For this review, take the finished solid that the model builds, in its own axes (mm). Face numbers are marked on the shaded views. A direction names the side the tool comes from. Coordinates: 2 decimals unless noted, no trailing zeros. Loops run counter-clockwise (first coordinate to the right, second up) from the corner with the lowest first, then second, coordinate; pieces in that order, holes last.
1. Mouldability with a two-part tool opening along X and no side actions: class the marked faces 4, 5, 6 and 7 as pulls with the +X half, pulls with the -X half, needs draft (parallel to the pull), parting line crosses it, or undercut.
2. Take a section at B-B, the plane z = -15.25. State the section outline as (x, y) points, then the cut area to 3 significant figures.
3. To check wall thickness, follow probe 1 along X at (y, z) = (0, -12); probe 2 along Z at (x, y) = (10.5, 2.25). State the ranges of each line that lie inside material, in increasing order.
4. Take a section at C-C, the plane y = -2.5. Count the separate pieces of the cut face and the enclosed holes in it, then the cut area to 3 significant figures.
5. Take a section at D-D, the plane z = -6. State the section outline as (x, y) points.
6. Take a section at A-A, the plane x = 0. State the section outline as (y, z) points.
7. Clearance check with flat-ended pins moving along their axes: P1, Ø3, axis at y = 6.5, z = -10, coming from the +X side; P2, Ø0.8, axis at x = 7, z = -9, coming from the +Y side; P3, Ø8, axis at x = 0, y = 0, coming from the +Z side. State where each tip first meets the part, or that it passes through.
8. Machinability: for the marked faces 1, 2 and 3, which of the approach directions +Z, -Z, +X, -X, +Y, -Y give a long, thin tool a straight path to every point of the face, cutting with its end or side? Answer none if there is none.
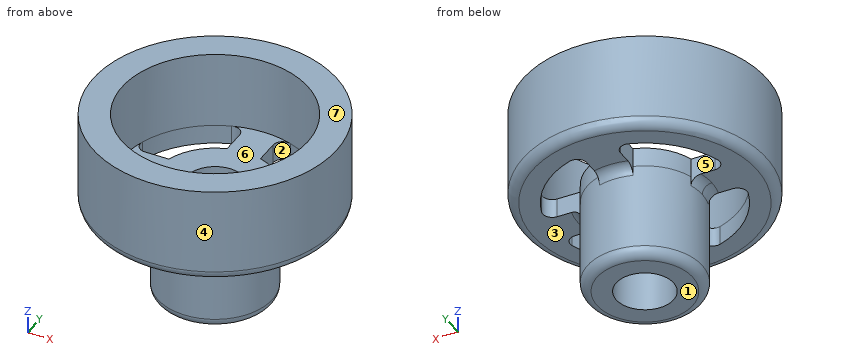
```python
from build123d import *
from build123d.topology import SkipClean

# Parameters (mm, degrees)
ESBO_O1_R                = 12.7
ESBO_O1_R_2              = 9.7
ESBO_O1_R_3              = 3
RESSALTO_EXTRUS_O1_DEPTH = 10
ESBO_O1_3_R              = 9.7
ESBO_O1_3_R_2            = 3
CORTE_EXTRUS_O1_DEPTH    = 8
CORTE_EXTRUS_O3_START    = -2
CORTE_EXTRUS_O3_DEPTH    = 2
FILETE1_R                = 1
ESBO_O2_5_R              = 6
ESBO_O2_5_R_2            = 3
RESSALTO_EXTRUS_O2_DEPTH = 10
FILETE2_R                = 1
FILETE3_R                = 1
FILETE4_R                = 1


with BuildPart() as part:
    # Esboço1 → Ressalto-extrusão1 (new body)
    # profile 1 of 2: a face of its own
    with BuildSketch(Plane.XY):
        Circle(ESBO_O1_R)
        Circle(ESBO_O1_R_2, mode=Mode.SUBTRACT)
    # profile 2 of 2: a face of its own
    with BuildSketch(Plane.XY):
        Circle(ESBO_O1_R_2)
        Circle(ESBO_O1_R_3, mode=Mode.SUBTRACT)
    extrude(amount=-RESSALTO_EXTRUS_O1_DEPTH)

    # Esboço1<3> → Corte-extrusão1 (cut)
    with BuildSketch(Plane.XY):
        Circle(ESBO_O1_3_R)
        Circle(ESBO_O1_3_R_2, mode=Mode.SUBTRACT)
    extrude(amount=-CORTE_EXTRUS_O1_DEPTH, mode=Mode.SUBTRACT)

    # Esboço2 → Corte-extrusão3 (cut)
    with SkipClean():  # the faces are left unmerged after this step: merging them gives an invalid solid
        with BuildSketch(Plane(origin=(0, 0, -10), x_dir=(-1, 0, 0), z_dir=(0, 0, -1)).offset(CORTE_EXTRUS_O3_START)):
            with BuildLine():
                Line((-1.75, -9.540833), (-1.75, -5.73912))
                ThreePointArc((-1.75, -5.73912), (-4.242641, -4.242641), (-5.73912, -1.75))
                Line((-5.73912, -1.75), (-9.540833, -1.75))
                ThreePointArc((-9.540833, -1.75), (-6.858936, -6.858936), (-1.75, -9.540833))
            make_face()
            with BuildLine():
                Line((-9.540833, 1.75), (-5.73912, 1.75))
                ThreePointArc((-5.73912, 1.75), (-4.242641, 4.242641), (-1.75, 5.73912))
                Line((-1.75, 5.73912), (-1.75, 9.540833))
                ThreePointArc((-1.75, 9.540833), (-6.858936, 6.858936), (-9.540833, 1.75))
            make_face()
            with BuildLine():
                Line((5.73912, 1.75), (9.540833, 1.75))
                ThreePointArc((9.540833, 1.75), (6.858936, 6.858936), (1.75, 9.540833))
                Line((1.75, 9.540833), (1.75, 5.73912))
                ThreePointArc((1.75, 5.73912), (4.242641, 4.242641), (5.73912, 1.75))
            make_face()
            with BuildLine():
                ThreePointArc((1.75, -9.540833), (6.858936, -6.858936), (9.540833, -1.75))
                Line((9.540833, -1.75), (5.73912, -1.75))
                ThreePointArc((5.73912, -1.75), (4.242641, -4.242641), (1.75, -5.73912))
                Line((1.75, -5.73912), (1.75, -9.540833))
            make_face()
        extrude(amount=CORTE_EXTRUS_O3_DEPTH, mode=Mode.SUBTRACT)

    # Filete1
    filete1_edges = [part.edges().sort_by_distance(p)[0] for p in [
        (-9.540833, -1.75, -9),
        (-1.75, -9.540833, -9),
        (-1.75, 9.540833, -9),
        (-9.540833, 1.75, -9),
        (9.540833, 1.75, -9),
        (1.75, 9.540833, -9),
        (1.75, -9.540833, -9),
        (9.540833, -1.75, -9),
    ]]
    fillet(filete1_edges, radius=FILETE1_R)

    # Esboço2<5> → Ressalto-extrusão2 (add)
    with SkipClean():  # the faces are left unmerged after this step: merging them gives an invalid solid
        with BuildSketch(Plane(origin=(0, 0, -10), x_dir=(-1, 0, 0), z_dir=(0, 0, -1))):
            Circle(ESBO_O2_5_R)
            with Locations(Location((0, 0, 0), (0, 0, 180))):
                Circle(ESBO_O2_5_R_2, mode=Mode.SUBTRACT)
        extrude(amount=RESSALTO_EXTRUS_O2_DEPTH)

    # Filete2
    # the kernel refuses this fillet: 1 mm, written as the material it adds along each edge
    with BuildSketch(Plane(origin=(0, 0, -10), x_dir=(-1, 0, 0), z_dir=(0, -1, 0))) as filete2_piece_1_section:
        with BuildLine():
            CenterArc((6 + FILETE2_R, FILETE2_R), FILETE2_R, 180, 90)
            Line((6, FILETE2_R), (6, 0))
            Line((6, 0), (6 + FILETE2_R, 0))
        make_face()
    filete2_piece_1 = revolve(axis=Axis((0, 0, -10), (0, 0, -1)), revolution_arc=40.831345, mode=Mode.PRIVATE)
    filete2_piece_1 = split(filete2_piece_1, bisect_by=Plane(origin=(-6.142197, 1.75, -10.226515), z_dir=(0, -1, 0)), keep=Keep.TOP, mode=Mode.PRIVATE)
    add(filete2_piece_1)
    with BuildSketch(Plane(origin=(0, 0, -10), x_dir=(0.6538481250913037, -0.7566258185619804, 0), z_dir=(0.7566258185619804, 0.6538481250913037, 0))) as filete2_piece_2_section:
        with BuildLine():
            CenterArc((6 + FILETE2_R, FILETE2_R), FILETE2_R, 180, 90)
            Line((6, FILETE2_R), (6, 0))
            Line((6, 0), (6 + FILETE2_R, 0))
        make_face()
    filete2_piece_2 = revolve(axis=Axis((0, 0, -10), (0, 0, -1)), revolution_arc=81.664733, mode=Mode.PRIVATE)
    filete2_piece_2 = split(filete2_piece_2, bisect_by=Plane(origin=(-1.75, -6.142197, -10.226515), z_dir=(1, 0, 0)), keep=Keep.TOP, mode=Mode.PRIVATE)
    filete2_piece_2 = split(filete2_piece_2, bisect_by=Plane(origin=(1.75, -6.142197, -10.226515), z_dir=(-1, 0, 0)), keep=Keep.TOP, mode=Mode.PRIVATE)
    add(filete2_piece_2)
    with BuildSketch(Plane(origin=(0, 0, -10), x_dir=(0.7566258185619548, 0.6538481250913332, 0), z_dir=(-0.6538481250913332, 0.7566258185619548, 0))) as filete2_piece_3_section:
        with BuildLine():
            CenterArc((6 + FILETE2_R, FILETE2_R), FILETE2_R, 180, 90)
            Line((6, FILETE2_R), (6, 0))
            Line((6, 0), (6 + FILETE2_R, 0))
        make_face()
    filete2_piece_3 = revolve(axis=Axis((0, 0, -10), (0, 0, -1)), revolution_arc=81.664733, mode=Mode.PRIVATE)
    filete2_piece_3 = split(filete2_piece_3, bisect_by=Plane(origin=(6.142197, -1.75, -10.226515), z_dir=(0, 1, 0)), keep=Keep.TOP, mode=Mode.PRIVATE)
    filete2_piece_3 = split(filete2_piece_3, bisect_by=Plane(origin=(6.142197, 1.75, -10.226515), z_dir=(0, -1, 0)), keep=Keep.TOP, mode=Mode.PRIVATE)
    add(filete2_piece_3)
    with BuildSketch(Plane(origin=(0, 0, -10), x_dir=(-0.6538481250913029, 0.7566258185619811, 0), z_dir=(-0.7566258185619811, -0.6538481250913029, 0))) as filete2_piece_4_section:
        with BuildLine():
            CenterArc((6 + FILETE2_R, FILETE2_R), FILETE2_R, 180, 90)
            Line((6, FILETE2_R), (6, 0))
            Line((6, 0), (6 + FILETE2_R, 0))
        make_face()
    filete2_piece_4 = revolve(axis=Axis((0, 0, -10), (0, 0, -1)), revolution_arc=81.664733, mode=Mode.PRIVATE)
    filete2_piece_4 = split(filete2_piece_4, bisect_by=Plane(origin=(1.75, 6.142197, -10.226515), z_dir=(-1, 0, 0)), keep=Keep.TOP, mode=Mode.PRIVATE)
    filete2_piece_4 = split(filete2_piece_4, bisect_by=Plane(origin=(-1.75, 6.142197, -10.226515), z_dir=(1, 0, 0)), keep=Keep.TOP, mode=Mode.PRIVATE)
    add(filete2_piece_4)
    with BuildSketch(Plane(origin=(0, 0, -10), x_dir=(-0.7566374717500711, -0.6538346399080277, 0), z_dir=(0.6538346399080277, -0.7566374717500711, 0))) as filete2_piece_5_section:
        with BuildLine():
            CenterArc((6 + FILETE2_R, FILETE2_R), FILETE2_R, 180, 90)
            Line((6, FILETE2_R), (6, 0))
            Line((6, 0), (6 + FILETE2_R, 0))
        make_face()
    filete2_piece_5 = revolve(axis=Axis((0, 0, -10), (0, 0, -1)), revolution_arc=40.831345, mode=Mode.PRIVATE)
    filete2_piece_5 = split(filete2_piece_5, bisect_by=Plane(origin=(-6.142196, -1.75, -10.226515), z_dir=(0, 1, 0)), keep=Keep.TOP, mode=Mode.PRIVATE)
    add(filete2_piece_5)

    # Filete3
    filete3_edges = [part.edges().sort_by_distance(p)[0] for p in [
        (6, 0, -20),
    ]]
    fillet(filete3_edges, radius=FILETE3_R)

    # Filete4
    filete4_edges = [part.edges().sort_by_distance(p)[0] for p in [
        (-12.7, 0, -10),
    ]]
    fillet(filete4_edges, radius=FILETE4_R)


solid = part.part
```
Results list:
1. face 4: parting line crosses it
1. face 5: undercut
1. face 6: undercut
1. face 7: needs draft
2. outline: circle Ø12 at (0, 0); hole circle Ø6 at (0, 0)
2. area: 84.8 mm2
3. probe 1: x = -6 to -3, 3 to 6
3. probe 2: z = -10 to 0
4. separate pieces: 4
4. enclosed holes: 0
4. area: 152 mm2
5. outline: circle Ø25.4 at (0, 0); hole circle Ø19.4 at (0, 0)
6. outline: (-12.7, -9) arc R1 ccw to (-11.7, -10) - (-7, -10) arc R1 cw to (-6, -11) - (-6, -19) arc R1 ccw to (-5, -20) - (-3, -20) - (-3, -8) - (-9.7, -8) - (-9.7, 0) - (-12.7, 0) - close; (3, -20) - (5, -20) arc R1 ccw to (6, -19) - (6, -11) arc R1 cw to (7, -10) - (11.7, -10) arc R1 ccw to (12.7, -9) - (12.7, 0) - (9.7, 0) - (9.7, -8) - (3, -8) - close
7. P1: stops at x = 11.55
7. P2: stops at y = 10.85
7. P3: stops at z = -8
8. face 1: -Z, +X, -X, +Y, -Y
8. face 2: +Z, -Z
8. face 3: -Z
